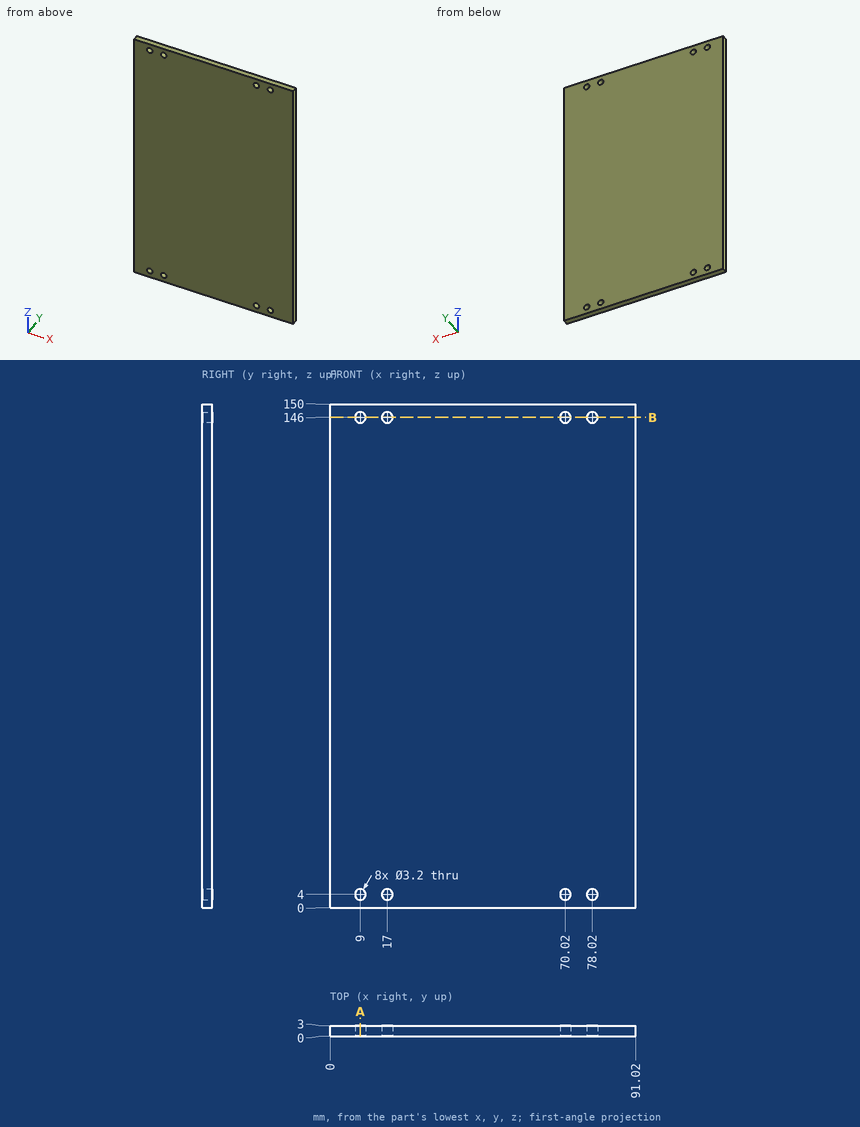
Geometry check sheet. Reference: drawing and pictorial views, mm from the part's lowest x, y, z. Coordinates: 2 decimals unless noted, no trailing zeros. Loops run counter-clockwise (first coordinate to the right, second up) from the corner with the lowest first, then second, coordinate; pieces in that order, holes last. Notation, with made-up numbers: (68, 29) -> (115, 29) arc R22 cw to (115, 50) -> close; hole circle Ø3 at (76.25, 9.5). An arc over 180 degrees is marked (long way). Write item = value, one per line. Start each with the question number.
1. Section check A-A on x = 9. Record the cut outline in (y, z), then the cut area to 3 significant figures.
2. Depth check by flat-ended pin: P1, Ø3.5, axis at x = 78.02, z = 146, coming from the -Y side. Enter the tip coordinate at first touch or a pass-through.
3. Material ranges on line 1 (X direction, y = 1.6, z = 146); line 2 (Z direction, x = 9, y = 2.4), recorded low to high.
4. Section check B-B on z = 146. Record the cut outline in (x, y).
Responses:
q1.outline = (0, 0) -> (3, 0) -> (3, 2.4) -> (0, 2.4) -> close; (0, 5.6) -> (3, 5.6) -> (3, 144.4) -> (0, 144.4) -> close; (0, 147.6) -> (3, 147.6) -> (3, 150) -> (0, 150) -> close
q1.area = 431 mm2
q2.P1 = 0
q3.line_1 = 0 to 7.4, 10.6 to 15.4, 18.6 to 68.42, 71.62 to 76.42, 79.62 to 91.02
q3.line_2 = 0 to 2.4, 5.6 to 144.4, 147.6 to 150
q4.outline = (0, 0) -> (7.4, 0) -> (7.4, 3) -> (0, 3) -> close; (10.6, 0) -> (15.4, 0) -> (15.4, 3) -> (10.6, 3) -> close; (18.6, 0) -> (68.42, 0) -> (68.42, 3) -> (18.6, 3) -> close; (71.62, 0) -> (76.42, 0) -> (76.42, 3) -> (71.62, 3) -> close; (79.62, 0) -> (91.02, 0) -> (91.02, 3) -> (79.62, 3) -> close
